Geometry: see drawing. Coordinates: mm, zero at the bounding-box minimum. A direction names the side the tool comes from. Coordinates: 2 decimals unless noted, no trailing zeros. Order: outer loops, then holes, each group sorted by start corner. A loop starts at its lowest first (then second) coordinate and runs counter-clockwise, first axis right, second up. Notation, with made-up numbers: M 69.5,77 L 117.5,77 A26 ccw 117.5,99 Z; hole C 28.5,11 d2. An arc over 180 degrees is marked long. Answer in a Markdown table with one row per item.
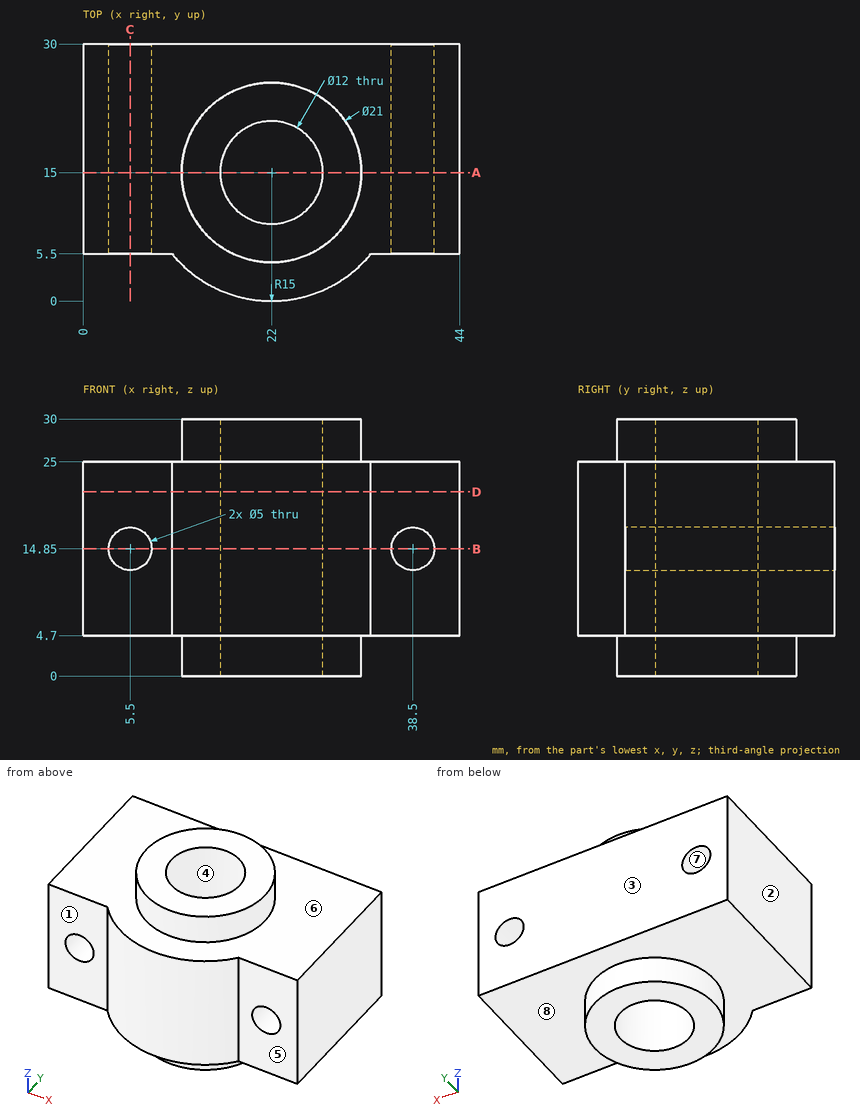
1) Contact query for flat-ended pins moving along their axis: pin 1 (5 mm diameter, centred on x = 25.5, z = 10, fed in from -Y); pin 2 (3 mm diameter, centred on x = 36.5, z = 17.5, fed in from -Y); pin 3 (3 mm diameter, centred on x = 38.5, z = 14.85, fed in from +Y); pin 4 (6 mm diameter, centred on x = 5.5, y = 26, fed in from +Z). Output: stop coordinate, or through.
Resolved:
| item | result |
|---|---|
| pin 1 | stops at y = 0.03 |
| pin 2 | stops at y = 5.5 |
| pin 3 | passes through |
| pin 4 | stops at z = 25 |
2) Mould query, pull axis Y, two halves, no side actions, for the marked faces 1, 2, 3 and 4. Classes: +Y half, -Y half, draft (parallel to the pull), parting line (faces both ways), or undercut.
Resolved:
| item | result |
|---|---|
| face 1 | -Y half |
| face 2 | draft |
| face 3 | +Y half |
| face 4 | undercut |
3) Cut plane C-C, the plane x = 5.5. Output: boundary loops of the cut face in (y, z).
Resolved:
| item | result |
|---|---|
| outline | M 5.5,4.7 L 30,4.7 L 30,12.35 L 5.5,12.35 Z; M 5.5,17.35 L 30,17.35 L 30,25 L 5.5,25 Z |
4) Material intervals for probe 1 along X at (y, z) = (27.5, 13.25); probe 2 along X at (y, z) = (21.5, 12.75); probe 3 along X at (y, z) = (14.25, 14.85), sorted ascending.
Resolved:
| item | result |
|---|---|
| probe 1 | x = 0 to 3.58, 7.42 to 36.58, 40.42 to 44 |
| probe 2 | x = 0 to 4.14, 6.86 to 37.14, 39.86 to 44 |
| probe 3 | x = 0 to 3, 8 to 16.05, 27.95 to 36, 41 to 44 |
5) Reachability of the marked faces 5, 6, 7 and 8 from +Z, -Z, +X, -X, +Y, -Y: full face, straight path, thin tool, end or side. Return the list, or none.
Resolved:
| item | result |
|---|---|
| face 5 | +Z, -Z, +X, -Y |
| face 6 | +Z |
| face 7 | +Y, -Y |
| face 8 | -Z |
6) Cut plane A-A, the plane y = 15. Output: boundary loops of the cut face in (x, z), and give its area (3 significant figures).
Resolved:
| item | result |
|---|---|
| outline | M 0,4.7 L 11.5,4.7 L 11.5,0 L 16,0 L 16,30 L 11.5,30 L 11.5,25 L 0,25 Z; M 28,0 L 32.5,0 L 32.5,4.7 L 44,4.7 L 44,25 L 32.5,25 L 32.5,30 L 28,30 Z; hole C 5.5,14.85 d5; hole C 38.5,14.85 d5 |
| area | 698 mm2 |
7) Cut plane B-B, the plane z = 14.85. Output: boundary loops of the cut face in (x, y).
Resolved:
| item | result |
|---|---|
| outline | M 0,5.5 L 3,5.5 L 3,30 L 0,30 Z; M 8,5.5 L 10.39,5.5 A15 ccw 33.61,5.5 L 36,5.5 L 36,30 L 8,30 Z; M 41,5.5 L 44,5.5 L 44,30 L 41,30 Z; hole C 22,15 d12 |
8) Cut plane D-D, the plane z = 21.5. Output: boundary loops of the cut face in (x, y), and give its area (3 significant figures).
Resolved:
| item | result |
|---|---|
| outline | M 0,5.5 L 10.39,5.5 A15 ccw 33.61,5.5 L 44,5.5 L 44,30 L 0,30 Z; hole C 22,15 d12 |
| area | 1,050 mm2 |
